from build123d import *

# Parameters (mm, degrees)
RESSALTO_EXTRUS_O1_DEPTH                             = 3
ESBO_O2_W                                            = 22
ESBO_O2_H                                            = 86.15
RESSALTO_EXTRUS_O2_DEPTH                             = 3
RESSALTO_EXTRUS_O3_DEPTH                             = 3
REBAIXO_PARA_SHCS_M21_D                              = 2.4
REBAIXO_PARA_SHCS_M21_DEPTH                          = 3
REBAIXO_PARA_SHCS_M21_CBORE_D                        = 4.4
REBAIXO_PARA_SHCS_M21_CBORE_DEPTH                    = 2
PADR_OCIRCULAR1_COUNT                                = 5
PADR_OCIRCULAR1_ANGLE                                = 180
ESBO_O10_R                                           = 2.75
RESSALTO_EXTRUS_O4_DEPTH                             = 0.6
REBAIXO_PARA_PARAFUSO_COM_CABE_A_PANELA_D            = 3.4
REBAIXO_PARA_PARAFUSO_COM_CABE_A_PANELA_CBORE_D      = 7
REBAIXO_PARA_PARAFUSO_COM_CABE_A_PANELA_CBORE_DEPTH  = 1.5
ESBO_O14_W                                           = 86.15
ESBO_O14_H                                           = 6
RESSALTO_EXTRUS_O5_DEPTH                             = 3
REBAIXO_PARA_PARAFUSO_COM_CABE_A_REDONDA_D           = 2.4
REBAIXO_PARA_PARAFUSO_COM_CABE_A_REDONDA_CBORE_D     = 4.4
REBAIXO_PARA_PARAFUSO_COM_CABE_A_REDONDA_CBORE_DEPTH = 1
FILETE2_R                                            = 3
FILETE1_R                                            = 3


with BuildPart() as part:
    # Esboço1 → Ressalto-extrusão1 (new body)
    with BuildSketch(Plane.XY):
        with BuildLine():
            Line((11, 0), (11, 23))
            Line((11, 23), (-11, 23))
            Line((-11, 23), (-11, 0))
            ThreePointArc((-11, 0), (-7.75, -3.25), (-4.5, 0))
            ThreePointArc((-4.5, 0), (0, 4.5), (4.5, 0))
            ThreePointArc((4.5, 0), (7.75, -3.25), (11, 0))
        make_face()
    extrude(amount=RESSALTO_EXTRUS_O1_DEPTH)

    # Esboço2 → Ressalto-extrusão2 (add)
    with BuildSketch(Plane(origin=(0, 23, 0), x_dir=(1, 0, 0), z_dir=(0, 1, 0))):
        with Locations((0, 40.075)):
            Rectangle(ESBO_O2_W, ESBO_O2_H)
    extrude(amount=RESSALTO_EXTRUS_O2_DEPTH)

    # Esboço3 → Ressalto-extrusão3 (add)
    with BuildSketch(Plane(origin=(0, 0, -80.15), x_dir=(-1, 0, 0), z_dir=(0, 0, -1))):
        with BuildLine():
            Line((-11, 0), (-11, 23))
            Line((-11, 23), (11, 23))
            Line((11, 23), (11, 0))
            ThreePointArc((11, 0), (0, -11), (-11, 0))
        make_face()
    extrude(amount=RESSALTO_EXTRUS_O3_DEPTH)

    # Rebaixo para SHCS M21
    with Locations(Plane.XY.offset(3)):
        with Locations((8, 0)):
            rebaixo_para_shcs_m21 = CounterBoreHole(REBAIXO_PARA_SHCS_M21_D / 2, REBAIXO_PARA_SHCS_M21_CBORE_D / 2, REBAIXO_PARA_SHCS_M21_CBORE_DEPTH, depth=REBAIXO_PARA_SHCS_M21_DEPTH)

    # PadrãoCircular1: Rebaixo para SHCS M21 ×5 about axis
    padr_ocircular1_axis = Axis((0, 0, 0), (0, 0, 1))
    for i in range(1, PADR_OCIRCULAR1_COUNT):
        add(rebaixo_para_shcs_m21.rotate(padr_ocircular1_axis, i * PADR_OCIRCULAR1_ANGLE / (PADR_OCIRCULAR1_COUNT - 1)), mode=Mode.SUBTRACT)

    # Esboço10 → Ressalto-extrusão4 (add)
    with BuildSketch(Plane.XY.offset(-80.15)):
        with Locations(Location((0, 0, 0), (0, 0, 180))):
            Circle(ESBO_O10_R)
    extrude(amount=RESSALTO_EXTRUS_O4_DEPTH)

    # Rebaixo para parafuso com cabeça panela de M31 (through all)
    with Locations(Plane(origin=(0, 0, -83.15), x_dir=(-1, 0, 0), z_dir=(0, 0, -1))):
        with Locations((0, 0)):
            CounterBoreHole(REBAIXO_PARA_PARAFUSO_COM_CABE_A_PANELA_D / 2, REBAIXO_PARA_PARAFUSO_COM_CABE_A_PANELA_CBORE_D / 2, REBAIXO_PARA_PARAFUSO_COM_CABE_A_PANELA_CBORE_DEPTH)

    # Esboço14 → Ressalto-extrusão5 (add)
    with BuildSketch(Plane.ZY.offset(11)):
        with Locations((-40.075, 23)):
            Rectangle(ESBO_O14_W, ESBO_O14_H)
    ressalto_extrus_o5 = extrude(amount=-RESSALTO_EXTRUS_O5_DEPTH)

    # Espelhar2: Ressalto-extrusão5 across plane
    add(ressalto_extrus_o5.mirror(Plane(origin=(0, 0, 0), x_dir=(0, 0, 1), z_dir=(1, 0, 0))))

    # Rebaixo para parafuso com cabeça redonda de M21 (through all)
    with Locations(Plane(origin=(0, 23, 0), x_dir=(-1, 0, 0), z_dir=(0, -1, 0))):
        with Locations((5.656854249, 64.236417264), (5.656854249, 52.922708765), (-5.656854249, 52.922708765), (-5.656854249, 64.236417264)):
            CounterBoreHole(REBAIXO_PARA_PARAFUSO_COM_CABE_A_REDONDA_D / 2, REBAIXO_PARA_PARAFUSO_COM_CABE_A_REDONDA_CBORE_D / 2, REBAIXO_PARA_PARAFUSO_COM_CABE_A_REDONDA_CBORE_DEPTH)

    # Filete2
    filete2_edges = [part.edges().sort_by_distance(p)[0] for p in [
        (-9.5, 20, -80.15),
        (-9.5, 20, 0),
        (9.5, 20, -80.15),
        (9.5, 20, 0),
    ]]
    fillet(filete2_edges, radius=FILETE2_R)

    # Filete1
    # the kernel refuses this fillet: 3 mm, written as the material it adds along each edge
    with BuildSketch(Plane(origin=(8, 23, -80.15), x_dir=(0, 0, 1), z_dir=(-1, 0, 0))) as filete1_piece_1:
        with BuildLine():
            CenterArc((FILETE1_R, -FILETE1_R), FILETE1_R, 90, 90)
            Line((0, -FILETE1_R), (0, 0))
            Line((0, 0), (FILETE1_R, 0))
        make_face()
    extrude(amount=16)
    with BuildSketch(Plane(origin=(-8, 23, 0), x_dir=(0, -1, 0), z_dir=(0, 0, -1))) as filete1_piece_2_section:
        with BuildLine():
            CenterArc((FILETE1_R, -FILETE1_R), FILETE1_R, 90, 90)
            Line((0, -FILETE1_R), (0, 0))
            Line((0, 0), (FILETE1_R, 0))
        make_face()
    filete1_piece_2 = extrude(amount=80.15, mode=Mode.PRIVATE)
    filete1_piece_2 = filete1_piece_2 - Plane(origin=(-5.656854249, 22.304141759, -52.922708765), x_dir=(-1, 0, 0), z_dir=(0, -1, 0)) * Cylinder(2.2, 173, mode=Mode.PRIVATE)
    filete1_piece_2 = filete1_piece_2 - Plane(origin=(-5.656854249, 22.304141759, -64.236417264), x_dir=(-1, 0, 0), z_dir=(0, -1, 0)) * Cylinder(2.2, 173, mode=Mode.PRIVATE)
    add(filete1_piece_2)
    with BuildSketch(Plane(origin=(8, 23, 0), x_dir=(0, 0, -1), z_dir=(-1, 0, 0))) as filete1_piece_3:
        with BuildLine():
            CenterArc((FILETE1_R, FILETE1_R), FILETE1_R, 180, 90)
            Line((0, FILETE1_R), (0, 0))
            Line((0, 0), (FILETE1_R, 0))
        make_face()
    extrude(amount=16)
    with BuildSketch(Plane(origin=(8, 23, 0), x_dir=(-1, 0, 0), z_dir=(0, 0, -1))) as filete1_piece_4_section:
        with BuildLine():
            CenterArc((FILETE1_R, -FILETE1_R), FILETE1_R, 90, 90)
            Line((0, -FILETE1_R), (0, 0))
            Line((0, 0), (FILETE1_R, 0))
        make_face()
    filete1_piece_4 = extrude(amount=80.15, mode=Mode.PRIVATE)
    filete1_piece_4 = filete1_piece_4 - Plane(origin=(5.656854249, 22.30418368, -52.922708765), x_dir=(-1, 0, 0), z_dir=(0, -1, 0)) * Cylinder(2.2, 173, mode=Mode.PRIVATE)
    filete1_piece_4 = filete1_piece_4 - Plane(origin=(5.656854249, 22.30418368, -64.236417264), x_dir=(-1, 0, 0), z_dir=(0, -1, 0)) * Cylinder(2.2, 173, mode=Mode.PRIVATE)
    add(filete1_piece_4)
    # the kernel refuses this fillet: 3 mm, written as the material it takes off along each edge
    with BuildSketch(Plane(origin=(-11, 26, -90.65), x_dir=(0, -1, 0), z_dir=(0, 0, 1)), Plane(origin=(11, 26, 10.5), x_dir=(0, -1, 0), z_dir=(0, 0, -1))) as filete1_2_piece_1:
        with BuildLine():
            CenterArc((FILETE1_R, FILETE1_R), FILETE1_R, 180, 90)
            Line((0, FILETE1_R), (0, 0))
            Line((0, 0), (FILETE1_R, 0))
        make_face()
    extrude(amount=101.15, mode=Mode.SUBTRACT)
    with BuildSketch(Plane(origin=(18.5, 26, 3), x_dir=(0, 0, -1), z_dir=(-1, 0, 0)), Plane(origin=(18.5, 26, -83.15), x_dir=(0, -1, 0), z_dir=(-1, 0, 0))) as filete1_2_piece_2:
        with BuildLine():
            CenterArc((FILETE1_R, FILETE1_R), FILETE1_R, 180, 90)
            Line((0, FILETE1_R), (0, 0))
            Line((0, 0), (FILETE1_R, 0))
        make_face()
    extrude(amount=37, mode=Mode.SUBTRACT)


solid = part.part
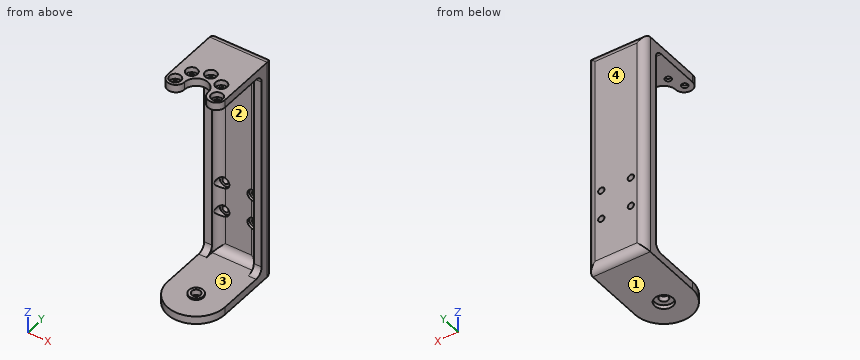
Design review of the part built by this model. Coordinates are the model's own, in mm. Face numbers are marked on the shaded views. A direction names the side the tool comes from. Give positions to 0.01 mm unless a question says otherwise; leave off trailing zeros. Loops run counter-clockwise (first coordinate to the right, second up) from the corner with the lowest first, then second, coordinate; pieces in that order, holes last. Notation, with made-up numbers: M 78.5,66 L 122.5,66 A24 ccw 122.5,78 Z; hole C 15.5,78.5 d1. An arc over 180 degrees is marked long. Answer as a JSON object with one key per item and string values.
Item 1: We need section C-C (y = -7.5). State the section outline as (x, z) points, and give its area (3 significant figures).
Output values:
{"outline": "M -8.05,-83.15 L 8.05,-83.15 L 8.05,-80.15 L -8.05,-80.15 Z", "area": "48.3 mm2"}
Item 2: Machinability: for the marked faces 3 and 4, which of the approach directions +Z, -Z, +X, -X, +Y, -Y give a long, thin tool a straight path to every point of the face, cutting with its end or side? Answer none if there is none.
Output values:
{"face 3": "none", "face 4": "+Z, -Z, +X, -X, +Y"}
Item 3: We need section A-A (y = 11.5). State the section outline as (x, z) points.
Output values:
{"outline": "M -11,-83.15 L 11,-83.15 L 11,-80.15 L -11,-80.15 Z; M -11,0 L 11,0 L 11,3 L -11,3 Z"}
Item 4: We need section B-B (z = -47). State the section outline as (x, y) points, and give its area (3 significant figures).
Output values:
{"outline": "M -11,20 L -8,20 A3 cw -5,23 L 5,23 A3 cw 8,20 L 11,20 L 11,23 A3 ccw 8,26 L -8,26 A3 ccw -11,23 Z", "area": "84.0 mm2"}
Item 5: Wall thickness on line 1 along Z through (x, y) = (-6, 13); line 2 along X through (y, z) = (8, 2.3); line 3 along Y through (x, z) = (2, -31): over which ranges is each line inside the solid? List them lowest first.
Output values:
{"line 1": "z = -83.15 to -80.15, 0 to 3", "line 2": "x = -11 to -2.2, 2.2 to 11", "line 3": "y = 23 to 26"}
Item 6: Mouldability with a two-part tool opening along X and no side actions: class the marked faces 1 and 2 as pulls with the +X half, pulls with the -X half, needs draft (parallel to the pull), parting line crosses it, or undercut.
Output values:
{"face 1": "needs draft", "face 2": "undercut"}
Item 7: For P1, Ø3.5, axis at x = 5, z = -54, coming from the -Y side; P2, Ø5, axis at x = 0, z = -31.5, coming from the -Y side; P3, Ø3, axis at x = -5.66, z = -64.24, coming from the -Y side, all flat-tipped, find the tip position at first contact; note any pin that passes through.
Output values:
{"P1": "stops at y = 22.62", "P2": "stops at y = 23", "P3": "stops at y = 24"}
